```python
from build123d import *

# Parameters (mm, degrees)
SKETCH1_W                                  = 708
SKETCH1_H                                  = 824
BOSS_EXTRUDE1_DEPTH                        = 5
SKETCH2_W                                  = 370
SKETCH2_H                                  = 500
CUT_EXTRUDE1_DEPTH                         = 3.5
SKETCH3_W                                  = 628
SKETCH3_H                                  = 500
CUT_EXTRUDE2_DEPTH                         = 2
SKETCH11_R                                 = 5.1
CUT_EXTRUDE7_DEPTH                         = 23.2
MIRROR4_AT_THE_SECOND_PLANE_COPY_1_SKETC_R = 5.1
MIRROR4_AT_THE_SECOND_PLANE_COPY_1_DEPTH   = 23.2
SKETCH4_R                                  = 10
CUT_EXTRUDE8_DEPTH                         = 1087.394150389


with BuildPart() as part:
    # Sketch1 → Boss-Extrude1 (new body)
    with BuildSketch(Plane(origin=(0, 0, 0), x_dir=(1, 0, 0), z_dir=(0, 1, 0))):
        with Locations((354, 412)):
            Rectangle(SKETCH1_W, SKETCH1_H)
    extrude(amount=BOSS_EXTRUDE1_DEPTH)

    # Sketch2 → Cut-Extrude1 (cut)
    with BuildSketch(Plane(origin=(0, 5, 0), x_dir=(1, 0, 0), z_dir=(0, 1, 0))):
        with Locations((354, 404)):
            Rectangle(SKETCH2_W, SKETCH2_H)
    extrude(amount=-CUT_EXTRUDE1_DEPTH, mode=Mode.SUBTRACT)

    # Sketch3 → Cut-Extrude2 (cut)
    with BuildSketch(Plane(origin=(0, 5, 0), x_dir=(1, 0, 0), z_dir=(0, 1, 0))):
        with Locations((354, 404)):
            Rectangle(SKETCH3_W, SKETCH3_H)
    extrude(amount=-CUT_EXTRUDE2_DEPTH, mode=Mode.SUBTRACT)

    # Sketch11 → Cut-Extrude7 (cut)
    with BuildSketch(Plane(origin=(0, 5, 0), x_dir=(1, 0, 0), z_dir=(0, 1, 0))):
        with Locations(Location((14, 14, 0), (0, 0, 270))):
            Circle(SKETCH11_R)
    cut_extrude7 = extrude(amount=-CUT_EXTRUDE7_DEPTH, mode=Mode.SUBTRACT)

    # Mirror4: Cut-Extrude7 across plane
    add(cut_extrude7.mirror(Plane(origin=(354, 0, 0), x_dir=(0, 0, 1), z_dir=(1, 0, 0))), mode=Mode.SUBTRACT)

    # Mirror4 at the second plane: Cut-Extrude7 across plane
    add(cut_extrude7.mirror(Plane.XY.offset(-412)), mode=Mode.SUBTRACT)

    # Mirror4 at the second plane copy 1 sketc → Mirror4 at the second plane copy 1 (cut)
    with BuildSketch(Plane(origin=(708, 5, -824), x_dir=(-1, 0, 0), z_dir=(0, 1, 0))):
        with Locations(Location((14, 14, 0), (0, 0, 270))):
            Circle(MIRROR4_AT_THE_SECOND_PLANE_COPY_1_SKETC_R)
    extrude(amount=-MIRROR4_AT_THE_SECOND_PLANE_COPY_1_DEPTH, mode=Mode.SUBTRACT)

    # Sketch4 → Cut-Extrude8 (cut, through all)
    with BuildSketch(Plane(origin=(0, 1.5, 0), x_dir=(1, 0, 0), z_dir=(0, 1, 0))):
        with Locations(Location((189, 634, 0), (0, 0, 270))):
            Circle(SKETCH4_R)
        with Locations(Location((319, 634, 0), (0, 0, 270))):
            Circle(SKETCH4_R)
        with Locations(Location((389, 634, 0), (0, 0, 270))):
            Circle(SKETCH4_R)
        with Locations(Location((519, 634, 0), (0, 0, 270))):
            Circle(SKETCH4_R)
        with Locations(Location((519, 174, 0), (0, 0, 90))):
            Circle(SKETCH4_R)
        with Locations(Location((389, 174, 0), (0, 0, 90))):
            Circle(SKETCH4_R)
        with Locations(Location((319, 174, 0), (0, 0, 90))):
            Circle(SKETCH4_R)
        with Locations(Location((189, 174, 0), (0, 0, 90))):
            Circle(SKETCH4_R)
    extrude(amount=-CUT_EXTRUDE8_DEPTH, mode=Mode.SUBTRACT)


solid = part.part
```
Design review of the part built by this model. Coordinates are the model's own, in mm. A direction names the side the tool comes from. Coordinates: 2 decimals unless noted, no trailing zeros. Write each loop counter-clockwise with the first axis right and the second up, starting at its lowest first coordinate (ties: lowest second). Pieces come first, ordered by that corner, then holes.
1) Add section D-D (x = 421). Write out the cut boundary in (y, z), plus the area to 3 significant figures.
2) Add section C-C (y = 4.15). Write out the cut boundary in (x, z), plus the area to 3 significant figures.
3) To check wall thickness, follow L1, parallel to Z at x = 694, y = 3.9; L2, parallel to X at y = 4, z = -14; L3, parallel to X at y = 0.3, z = -634. State the ranges of each line that lie inside material, in increasing order.
4) Mouldability with a two-part tool opening along X and no side actions: class faces 3 (the flat face through (34, 5, -418)), 4 (the cylindrical face through (527.43, 0.76, -628.62)) as +X half, -X half, draft (parallel to the pull), parting line (faces both ways), or undercut.
5) Add section A-A (z = -634). Write out the cut boundary in (x, y), plus the area to 3 significant figures.
6) Machinability: for faces 1 (the flat face through (351, 1.5, -408)), 2 (the cylindrical face through (379.085, 0.76, -172.698)), which of the approach directions +Z, -Z, +X, -X, +Y, -Y give a long, thin tool a straight path to every point of the face, cutting with its end or side? Answer none if there is none.
7) Add section B-B (x = 519). Write out the cut boundary in (y, z), plus the area to 3 significant figures.
8) Insertion check: pin 1 (2 mm diameter, centred on x = 128.5, z = -254, fed in from +Y); pin 2 (23 mm diameter, centred on x = 189, z = -174, fed in from +Y). Each pin has a flat end and moves straight along its axis. Give the tip position at first contact, or say it passes through.
Check result:
1. outline: (0, -824) - (5, -824) - (5, -654) - (1.5, -654) - (1.5, -154) - (5, -154) - (5, 0) - (0, 0) - close
1. area: 2,370 mm2
2. outline: (0, -824) - (708, -824) - (708, 0) - (0, 0) - close; hole circle Ø10.2 at (14, -810); hole circle Ø10.2 at (14, -14); hole (40, -654) - (668, -654) - (668, -154) - (40, -154) - close; hole circle Ø10.2 at (694, -810); hole circle Ø10.2 at (694, -14)
2. area: 269,000 mm2
3. L1: z = -824 to -815.1, -804.9 to -19.1, -8.9 to 0
3. L2: x = 0 to 8.9, 19.1 to 688.9, 699.1 to 708
3. L3: x = 0 to 179, 199 to 309, 329 to 379, 399 to 509, 529 to 708
4. face 3: draft
4. face 4: undercut
5. outline: (0, 0) - (179, 0) - (179, 1.5) - (169, 1.5) - (169, 3) - (40, 3) - (40, 5) - (0, 5) - close; (199, 0) - (309, 0) - (309, 1.5) - (199, 1.5) - close; (329, 0) - (379, 0) - (379, 1.5) - (329, 1.5) - close; (399, 0) - (509, 0) - (509, 1.5) - (399, 1.5) - close; (529, 0) - (708, 0) - (708, 5) - (668, 5) - (668, 3) - (539, 3) - (539, 1.5) - (529, 1.5) - close
5. area: 1,610 mm2
6. face 1: +Y
6. face 2: +Y, -Y
7. outline: (0, -824) - (5, -824) - (5, -654) - (1.5, -654) - (1.5, -644) - (0, -644) - close; (0, -624) - (1.5, -624) - (1.5, -184) - (0, -184) - close; (0, -164) - (1.5, -164) - (1.5, -154) - (5, -154) - (5, 0) - (0, 0) - close
7. area: 2,310 mm2
8. pin 1: stops at y = 3
8. pin 2: stops at y = 1.5
